Could you check a few things on this model? Use its own coordinates, in mm. Give positions to 0.01 mm unless a question says otherwise; leave off trailing zeros. Write each loop counter-clockwise with the first axis right and the second up, starting at its lowest first coordinate (ties: lowest second). Pieces come first, ordered by that corner, then holes. Notation, with made-up numbers: (22.5, -21.75) - (30.5, -21.75) arc R19 ccw to (30.5, 9.25) - close; hole circle Ø7 at (77, 29.25). An arc over 180 degrees is marked (long way). Answer as CSV lines item,"result". Start each with the question number.
Q1. Will this pin go through, and if not, where does the flat tip stop? pin 1 Ø1 at (y, z) = (1.5, -1.5) entering from -X.
Q2. If I drill on line 1 along Y through (x, z) = (0, 0); line 2 along X through (y, z) = (0, -9); line 3 along X through (y, z) = (-1.9, 4), over which ranges is the centre line in solid material (lowest first)?
Q3. Imagine slicing it at A-A on z = -10. List the corners of the cut face in (x, y) for me.
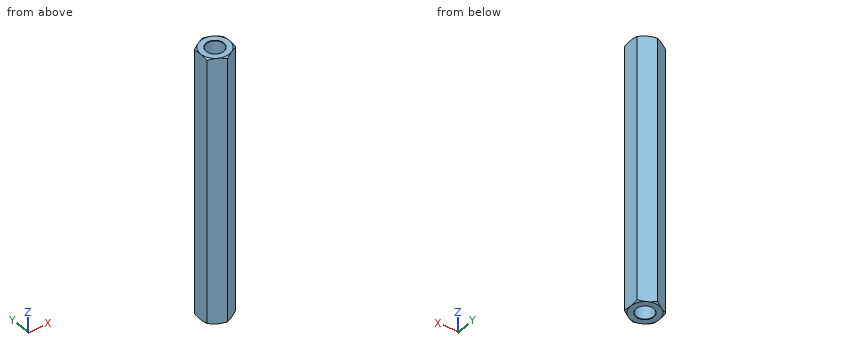
```python
from build123d import *

# Parameters (mm, degrees)
EXTRUDE1_DEPTH          = 22.225
EXTRUDE1_DEPTH_BACK     = 22.225
SKETCH1_R               = 1.4224
SKETCH8_OUTSIDE_W       = 173.728
SKETCH8_OUTSIDE_H       = 174.466
SKETCH8_OUTSIDE_R       = 2.38125
EXTRUDE4_DEPTH          = 45.598579802
EXTRUDE4_DRAFT          = -60
MIRROR1_COPY_1_SKETCH_W = 173.728
MIRROR1_COPY_1_SKETCH_H = 174.466
MIRROR1_COPY_1_SKETCH_R = 2.38125
MIRROR1_COPY_1_DEPTH    = 45.598579802
MIRROR1_COPY_1_DRAFT    = -60


with BuildPart() as part:
    # Sketch1 → Extrude1 (new, two sides: drawn at the far end of the back side and taken through both)
    with BuildSketch(Plane.XY.offset(-EXTRUDE1_DEPTH_BACK)):
        Polygon((0, 2.749630657), (-2.38125, 1.374815329), (-2.38125, -1.374815329), (0, -2.749630657), (2.38125, -1.374815329), (2.38125, 1.374815329), align=None)
        Circle(SKETCH1_R, mode=Mode.SUBTRACT)
    extrude(amount=EXTRUDE1_DEPTH + EXTRUDE1_DEPTH_BACK)

    # Extrude3 cone 1 section (through the dimple's axis) → Extrude3 (revolve, cut)
    with BuildSketch(Plane(origin=(0, 0, -22.225), x_dir=(0, 1, 0), z_dir=(1, 0, 0))):
        Polygon((0, 0), (1.4732, 0), (0, 1.579813584), align=None)
    extrude3 = revolve(axis=Axis((0, 0, -22.225), (0, 0, 1)), mode=Mode.SUBTRACT)


with BuildPart() as extrude4_tool:
    # Sketch8 outside → Extrude4 (with draft: the straight prism first)
    with BuildSketch(Plane(origin=(0, 0, -22.225), x_dir=(-1, 0, 0), z_dir=(0, 0, -1))):
        Rectangle(SKETCH8_OUTSIDE_W, SKETCH8_OUTSIDE_H)
        Circle(SKETCH8_OUTSIDE_R, mode=Mode.SUBTRACT)
    extrude(amount=-EXTRUDE4_DEPTH)
    # Extrude4: the draft: its side faces are tilted about the plane it starts from
    extrude4_sides = [extrude4_tool.faces().sort_by_distance(p)[0] for p in [
        (0, -87.233, 0.574289901),
        (-86.864, 0, 0.574289901),
        (0, 87.233, 0.574289901),
        (86.864, 0, 0.574289901),
        (2.38125, 0, 0.574289901),
    ]]
    draft(extrude4_sides, Plane(origin=(0, 0, -22.225), x_dir=(-1, 0, 0), z_dir=(0, 0, -1)), EXTRUDE4_DRAFT)


with BuildPart() as part_1:
    add(part.part)

    # Extrude4: cut by extrude4_tool
    add(extrude4_tool.part, mode=Mode.SUBTRACT)

    # Mirror1: Extrude3 across plane
    add(extrude3.mirror(Plane.XY), mode=Mode.SUBTRACT)


with BuildPart() as mirror1_copy_1_tool:
    # Mirror1 copy 1 sketch → Mirror1 copy 1 (with draft: the straight prism first)
    with BuildSketch(Plane(origin=(0, 0, 22.225), x_dir=(-1, 0, 0), z_dir=(0, 0, 1))):
        Rectangle(MIRROR1_COPY_1_SKETCH_W, MIRROR1_COPY_1_SKETCH_H)
        Circle(MIRROR1_COPY_1_SKETCH_R, mode=Mode.SUBTRACT)
    extrude(amount=-MIRROR1_COPY_1_DEPTH)
    # Mirror1 copy 1: the draft: its side faces are tilted about the plane it starts from
    mirror1_copy_1_sides = [mirror1_copy_1_tool.faces().sort_by_distance(p)[0] for p in [
        (0, -87.233, -0.574289901),
        (-86.864, 0, -0.574289901),
        (0, 87.233, -0.574289901),
        (86.864, 0, -0.574289901),
        (2.38125, 0, -0.574289901),
    ]]
    draft(mirror1_copy_1_sides, Plane(origin=(0, 0, 22.225), x_dir=(-1, 0, 0), z_dir=(0, 0, 1)), MIRROR1_COPY_1_DRAFT)


with BuildPart() as part_2:
    add(part_1.part)

    # Mirror1 copy 1: cut by mirror1_copy_1_tool
    add(mirror1_copy_1_tool.part, mode=Mode.SUBTRACT)


solid = part_2.part
```
Conclusion:
1,pin 1,"x = -2.38"
2,line 1,"-2.75 to -1.42, 1.42 to 2.75"
2,line 2,"-2.38 to -1.42, 1.42 to 2.38"
2,line 3,"-1.47 to 1.47"
3,outline,"(-2.38, -1.37) - (0, -2.75) - (2.38, -1.37) - (2.38, 1.37) - (0, 2.75) - (-2.38, 1.37) - close; hole circle Ø2.84 at (0, 0)"
